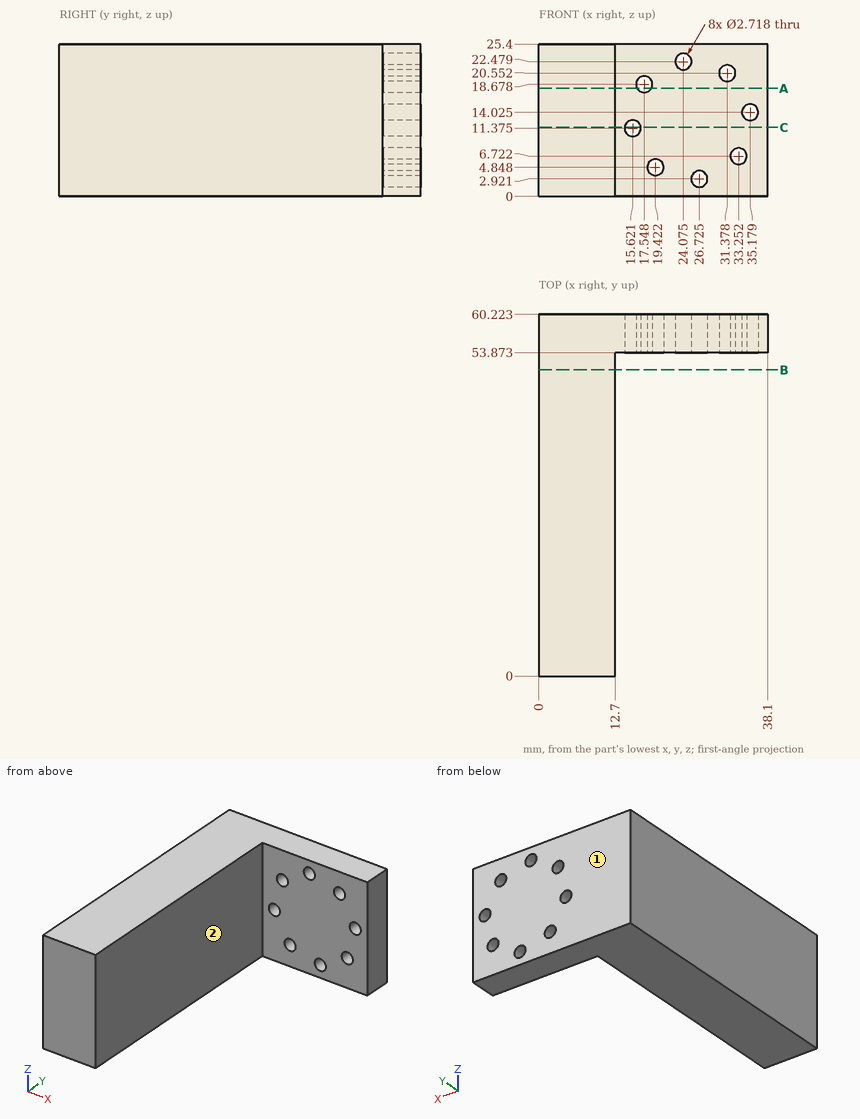
For this review, use the dimensioned drawing (mm, ordinates from the lowest corner) and the shaded views. A direction names the side the tool comes from. Round coordinates to 2 decimals unless told otherwise and drop trailing zeros. Order: outer loops, then holes, each group sorted by start corner. A loop starts at its lowest first (then second) coordinate and runs counter-clockwise, first axis right, second up. Notation, with made-up numbers: M 60.25,70 L 85.25,70 A14 cw 85.25,78 Z; hole C 59.5,-7 d8. An arc over 180 degrees is marked long. Write each question's results on one line, items separated by ' | '. Start each with the question number.
1. Add section C-C (z = 11.5). State the section outline as (x, y) points, then the cut area to 3 significant figures.
2. Add section A-A (z = 18). State the section outline as (x, y) points.
3. Add section B-B (y = 51). State the section outline as (x, z) points.
4. Tool access review of the marked faces 1 and 2: name each direction out of +Z, -Z, +X, -X, +Y, -Y from which nothing blocks a thin tool from reaching the whole face with its end or side.
5. Clearance check with flat-ended pins moving along their axes: pin 1 Ø4.5 at (x, z) = (19.42, 4.85) entering from -Y; pin 2 Ø2.5 at (x, z) = (33.25, 6.72) entering from -Y. State where each tip first meets the part, or that it passes through.
6. To check wall thickness, follow L1, parallel to Z at x = 16.5, y = 56.5 (1 decimal); L2, parallel to X at y = 51, z = 6.75; L3, parallel to Y at x = 29.5, z = 24.25. State the ranges of each line that lie inside material, in increasing order. Write a range as [from, to].
Output values:
1) outline: M 0,0 L 12.7,0 L 12.7,53.87 L 14.27,53.87 L 14.27,60.22 L 0,60.22 Z; M 16.97,53.87 L 38.1,53.87 L 38.1,60.22 L 16.97,60.22 Z | area: 909 mm^2
2) outline: M 0,0 L 12.7,0 L 12.7,53.87 L 16.37,53.87 L 16.37,60.22 L 0,60.22 Z; M 18.73,53.87 L 38.1,53.87 L 38.1,60.22 L 18.73,60.22 Z
3) outline: M 0,0 L 12.7,0 L 12.7,25.4 L 0,25.4 Z
4) face 1: +Z, -Z, +X, -X, +Y | face 2: +Z, -Z, +X, -Y
5) pin 1: y = 53.87 | pin 2: through
6) L1: [0, 10.3], [12.4, 17.8], [19.5, 25.4] | L2: [0, 12.7] | L3: [53.87, 60.22]
